Build history of the part. All positions in model axes, mm. Coordinates: 2 decimals unless noted, no trailing zeros. Write each loop counter-clockwise with the first axis right and the second up, starting at its lowest first coordinate (ties: lowest second). Pieces come first, ordered by that corner, then holes. Notation, with made-up numbers: (71, 35.25) -> (105, 35.25) arc R25 cw to (105, 67.25) -> close; hole circle Ø1 at (-35.75, 51). An arc over 180 degrees is marked (long way). Write each question's results on one line, items separated by ' | '. Start each with the question number.
Q1. Saw through at B-B on z = 0. Give the cut face in (x, y), and give its area (3 significant figures).
Q2. Saw through at C-C on x = -13. Give the cut face in (y, z).
Q3. Drill centre lines: line 1 (Y direction, x = 43, z = -22); line 2 (X direction, y = 132, z = 1); line 3 (Y direction, x = 3.5, z = -29.5). Where is each one in solid material? Low to high.
Q4. Drop flat-ended pins along their axis: pin 1 Ø3 at (x, y) = (35.5, 177) entering from -Z; pin 2 Ø5 at (x, y) = (-12, 162) entering from +Z; pin 3 Ø1.5 at (y, z) = (228, -19.5) entering from -X. Give the stop position or say it passes through.
Q5. Saw through at A-A on y = 63.5. Give the cut face in (x, z).
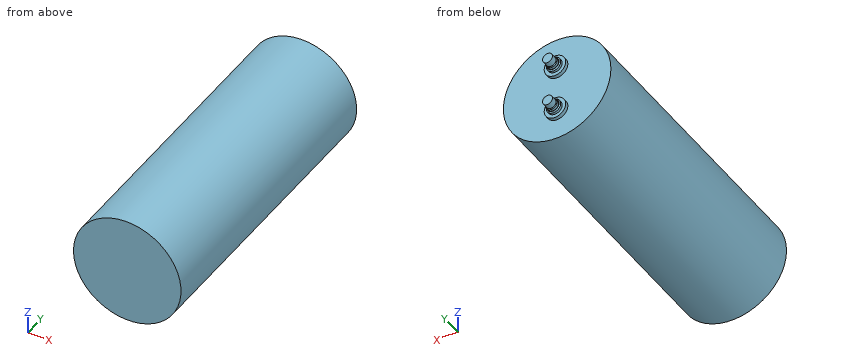
Autodesk Inventor part; units mm, degrees
ref_plane "YZ Plane" through (0, 0, 0) normal (1, 0, 0) x (0, 1, 0)
ref_plane "XZ Plane" through (0, 0, 0) normal (0, 1, 0) x (-1, 0, 0)
ref_plane "XY Plane" through (0, 0, 0) normal (0, 0, 1) x (1, 0, 0)
sketch "Sketch1" plane through (0, 0, 0) normal (0, 1, 0) x (-1, 0, 0)
  circle A0 centre (0, 0) radius 49.9618
  dimension "Diameter" = 99.9236
extrude "Extrusion1" add sketch "Sketch1" along normal blind 270
sketch "Sketch2" plane through (0, 270, 0) normal (0, 1, 0) x (1, 0, 0)
  circle A0 centre (0, -21.3551) radius 9.9758
  circle A1 centre (0, 21.3551) radius 9.9758
  line L0 (0, -21.3551) -> (0, 21.3551) construction
  point P0 (0, 0)
  point P1 (0, 0)
  dimension "d3" = 19.9517
  dimension "d6" = 42.7101
extrude "Extrusion2" add sketch "Sketch2" along normal blind 3.3528
sketch "Sketch3" plane through (0, 273.3528, 21.3551) normal (0, 1, 0) x (1, 0, 0)
  circle A0 centre (0, 42.7101) radius 9.9758 construction
  circle A1 centre (0, 0) radius 9.9758 construction
  circle A2 centre (0, 42.7101) radius 6.731
  circle A3 centre (0, 0) radius 6.731
  point P0 (0, 21.3551)
  dimension "d7" = 13.462
extrude "Extrusion3" add sketch "Sketch3" along normal blind 3.175
sketch "Sketch4" plane through (0, 276.5278, 21.3551) normal (0, 1, 0) x (1, 0, 0)
  circle A0 centre (0, 42.7101) radius 6.731 construction
  circle A1 centre (0, 0) radius 6.731 construction
  circle A2 centre (0, 42.7101) radius 5.4229
  circle A3 centre (0, 0) radius 5.4229
  point P0 (0, 21.3551)
  dimension "d10" = 10.8458
extrude "Extrusion4" add sketch "Sketch4" along normal blind 2.794
sketch "Sketch5" plane through (0, 279.3218, 21.3551) normal (0, 1, 0) x (1, 0, 0)
  circle A0 centre (0, 42.7101) radius 5.4229 construction
  circle A1 centre (0, 0) radius 5.4229 construction
  circle A2 centre (0, 42.7101) radius 4.6164
  circle A3 centre (0, 0) radius 4.6164
  point P0 (0, 21.3551)
  dimension "d13" = 9.2329
extrude "Extrusion5" add sketch "Sketch5" along normal blind 5.4864
thread "Thread1"
thread "Thread2"
chamfer "Chamfer1" distance 0.9525 angle 45 2 edges at (-6.731, 276.5278, -21.3551) (-6.731, 276.5278, 21.3551)
chamfer "Chamfer2" distance 0.6223 angle 45 2 edges at (-5.4229, 279.3218, 21.3551) (-5.4229, 279.3218, -21.3551)
properties part number "3.5F_Cap" material "Aluminum 6061"
Returned:
1) outline: (-49.96, 0) -> (49.96, 0) -> (49.96, 270) -> (-49.96, 270) -> close | area: 27,000 mm2
2) outline: (0, -48.24) -> (270, -48.24) -> (270, 48.24) -> (0, 48.24) -> close
3) line 1: y = 0 to 270 | line 2: x = -49.95 to 49.95 | line 3: y = 0 to 273.35
4) pin 1: stops at z = -36.61 | pin 2: stops at z = 49.05 | pin 3: stops at x = -46.31
5) outline: circle Ø99.92 at (0, 0)
